Part print with two shaded views. Sizes in mm from the minimum x, y, z corner. Coordinates: 2 decimals unless noted, no trailing zeros. Loops run counter-clockwise (first coordinate to the right, second up) from the corner with the lowest first, then second, coordinate; pieces in that order, holes last.
Item 1: Cut at B-B (x = 20). List the corners of the cut face in (y, z), and give its area (3 significant figures).
Item 2: Drill centre lines: line 1 along X through (y, z) = (24, 9) (1 decimal); line 2 along Z through (x, y) = (13.5, 15.5); line 3 along X through (y, z) = (30.5, 2). Where is each one in solid material? Low to high.
Item 3: Cut at C-C (x = 10). List the corners of the cut face in (y, z).
Item 4: Mould opens along Y. For the marked faces 1, 2, 3 and 4 say: released by +Y, released by -Y, zero draft, split by the parting line, or undercut.
Item 5: Flat gauge pins, fed straight in: pin 1 (24.5 mm diameter, centred on x = 23.495, y = 23.495, fed in from -Z); pin 2 (9 mm diameter, centred on x = 24, y = 17.5, fed in from -Z); pin 3 (3 mm diameter, centred on x = 23.5, y = 4.13, fed in from -Z); pin 4 (2 mm diameter, centred on x = 14, z = 20.5, fed in from -Y). Where does each tip first touch, or does it go through?
Item 6: Cut at D-D (z = 26). List the corners of the cut face in (x, y) (1 decimal), and give its area (3 significant figures).
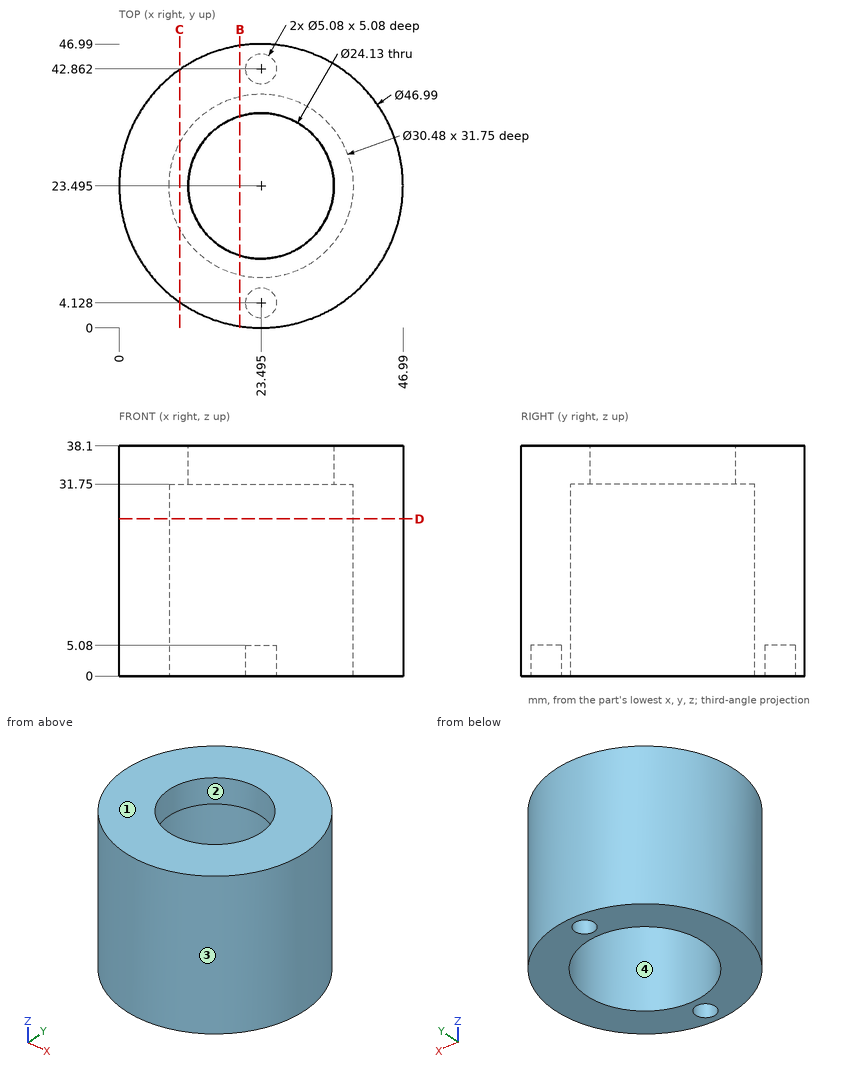
Filled sheet:
1. outline: (0.26, 0) - (8.66, 0) - (8.66, 31.75) - (11.95, 31.75) - (11.95, 38.1) - (0.26, 38.1) - close; (35.04, 31.75) - (38.33, 31.75) - (38.33, 0) - (46.73, 0) - (46.73, 38.1) - (35.04, 38.1) - close
1. area: 682 mm2
2. line 1: x = 0 to 8.3, 38.7 to 47
2. line 2: z = 31.75 to 38.1
2. line 3: x = 1.07 to 9.96, 37.03 to 45.92
3. outline: (4.26, 0) - (16.41, 0) - (16.41, 31.75) - (30.58, 31.75) - (30.58, 0) - (42.73, 0) - (42.73, 38.1) - (4.26, 38.1) - close
4. face 1: zero draft
4. face 2: undercut
4. face 3: split by the parting line
4. face 4: undercut
5. pin 1: stops at z = 31.75
5. pin 2: passes through
5. pin 3: stops at z = 5.08
5. pin 4: stops at y = 1.59
6. outline: circle Ø47 at (23.5, 23.5); hole circle Ø30.5 at (23.5, 23.5)
6. area: 1,000 mm2
